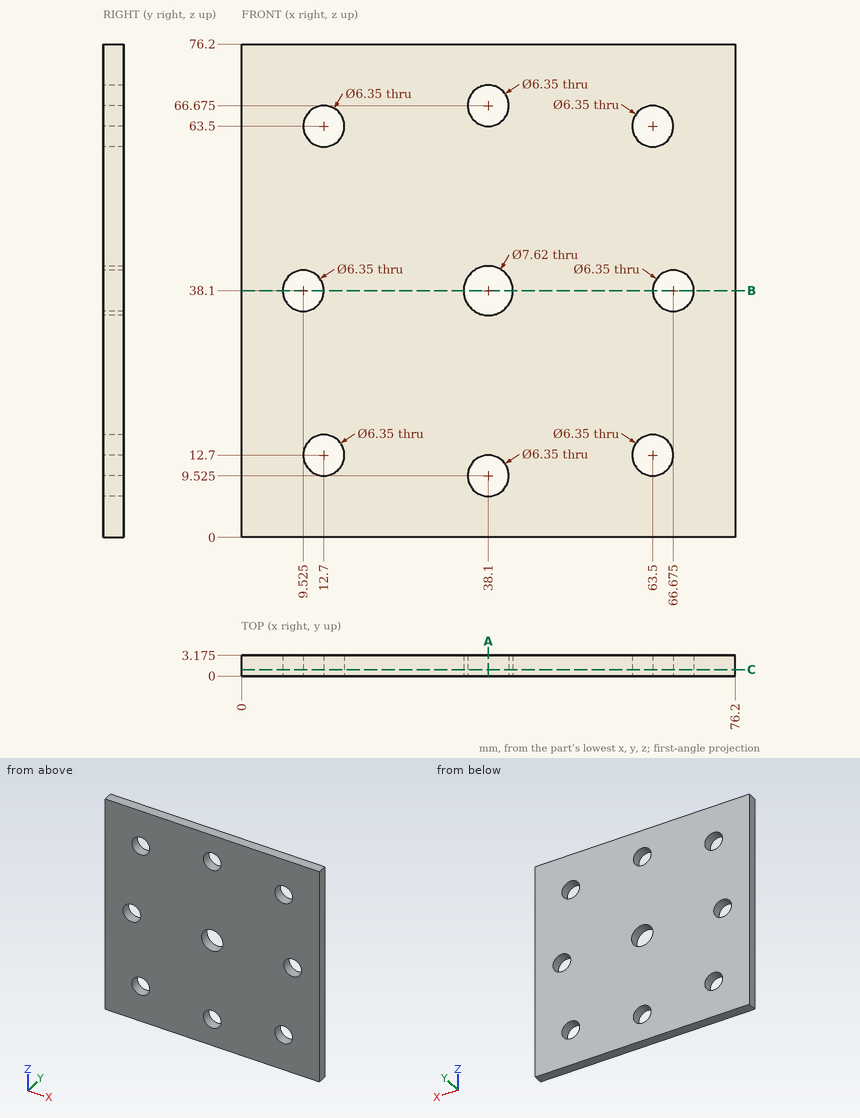
The drawing under review shows one solid part. Ordinate dimensions are in mm from its lowest x, y, z. Round coordinates to 2 decimals unless told otherwise and drop trailing zeros. Write each loop counter-clockwise with the first axis right and the second up, starting at its lowest first coordinate (ties: lowest second). Pieces come first, ordered by that corner, then holes. Notation, with made-up numbers: (77, 42) - (123, 42) arc R31 ccw to (123, 81) - close; hole circle Ø5 at (-27, -29.5). An arc over 180 degrees is marked (long way). One line per question, with ' | ' between items.
Item 1: Add section B-B, the plane z = 38.1. Give the boundary of the cut face in (x, y) (3 decimals), then the cut area to 3 significant figures.
Resolved:
outline: (0, 0) - (6.35, 0) - (6.35, 3.175) - (0, 3.175) - close; (12.7, 0) - (34.29, 0) - (34.29, 3.175) - (12.7, 3.175) - close; (41.91, 0) - (63.5, 0) - (63.5, 3.175) - (41.91, 3.175) - close; (69.85, 0) - (76.2, 0) - (76.2, 3.175) - (69.85, 3.175) - close | area: 177 mm2
Item 2: To check wall thickness, follow probe 1 along X at (y, z) = (0.75, 38.1); probe 2 along Z at (x, y) = (61, 2). State the ranges of each line that lie inside material, in increasing order.
Resolved:
probe 1: x = 0 to 6.35, 12.7 to 34.29, 41.91 to 63.5, 69.85 to 76.2 | probe 2: z = 0 to 10.74, 14.66 to 61.54, 65.46 to 76.2
Item 3: Add section C-C, the plane y = 1. State how many separate pieces and enclosed holes the cut face has, then the cut area to 3 significant figures.
Resolved:
separate pieces: 1 | enclosed holes: 9 | area: 5,510 mm2
Item 4: Add section A-A, the plane x = 38.1. Give the boundary of the cut face in (y, z) (3 decimals), then the cut area to 3 significant figures.
Resolved:
outline: (0, 0) - (3.175, 0) - (3.175, 6.35) - (0, 6.35) - close; (0, 12.7) - (3.175, 12.7) - (3.175, 34.29) - (0, 34.29) - close; (0, 41.91) - (3.175, 41.91) - (3.175, 63.5) - (0, 63.5) - close; (0, 69.85) - (3.175, 69.85) - (3.175, 76.2) - (0, 76.2) - close | area: 177 mm2
